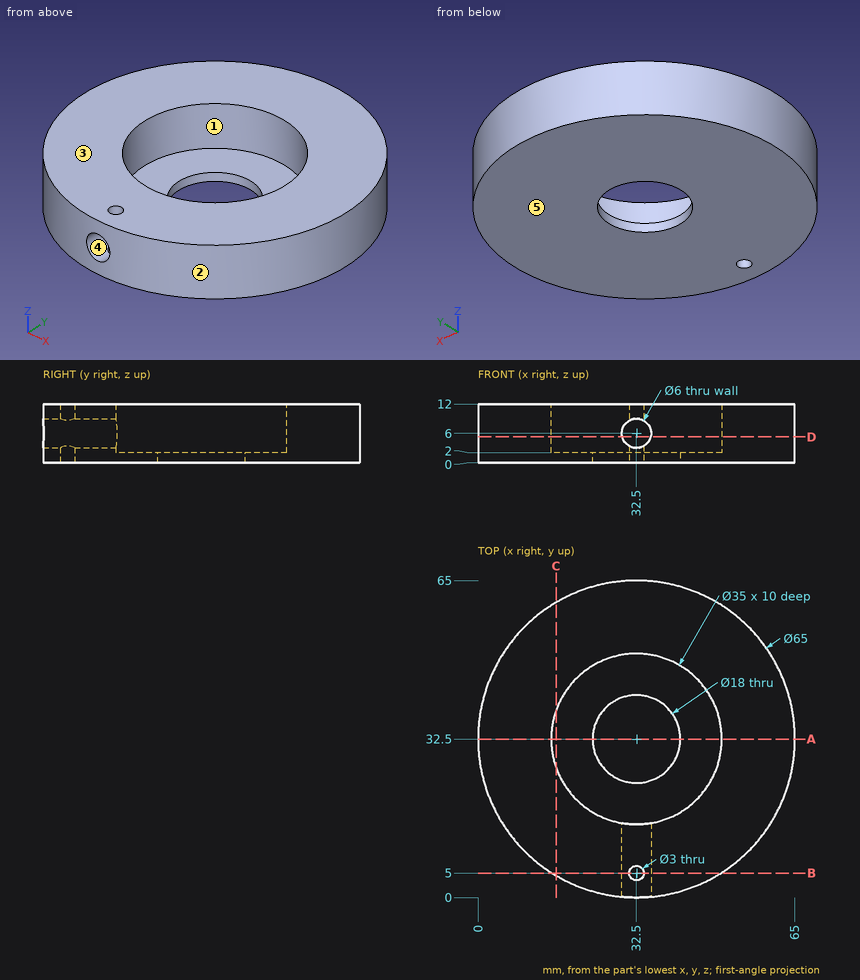
Could you check a few things on this drawing? It's one solid part, dimensions in mm from its lowest x, y, z. A direction names the side the tool comes from. Coordinates: 2 decimals unless noted, no trailing zeros. Write each loop counter-clockwise with the first axis right and the second up, starting at its lowest first coordinate (ties: lowest second). Pieces come first, ordered by that corner, then holes.
1) Thinking about a two-plate mould opening in Z: for the marked faces 3, 4 and 5, which applies, +Z half, -Z half, draft (parallel to the pull), parting line (faces both ways), or undercut?
Filled in:
face 3: +Z half
face 4: undercut
face 5: -Z half
2) Which directions (+Z, -Z, +X, -X, +Y, -Y) give clear straight access to the entire face, cutting with the end or side of a thin tool? Please do the marked faces 1 and 2.
Filled in:
face 1: +Z
face 2: +Z, -Z
3) If we section it at A-A (y = 32.5): List the corners of the cut face in (x, z) for me, plus the area to 3 significant figures.
Filled in:
outline: (0, 0) - (23.5, 0) - (23.5, 2) - (15, 2) - (15, 12) - (0, 12) - close; (41.5, 0) - (65, 0) - (65, 12) - (50, 12) - (50, 2) - (41.5, 2) - close
area: 394 mm2
4) If we section it at D-D (z = 5.25): List the corners of the cut face in (x, y) for me.
Filled in:
outline: (29.6, 0.13) - (29.6, 15.24) arc R17.5 cw (long way) to (35.4, 15.24) - (35.4, 0.13) arc R32.5 ccw (long way) to start
5) I'm going to push flat-ended pins straight in: pin 1 (4 mm diameter, centred on x = 32.5, y = 5, fed in from +Z); pin 2 (5 mm diameter, centred on x = 32.5, z = 6, fed in from +Y); pin 3 (2.5 mm diameter, centred on x = 32.5, y = 5, fed in from +Z); pin 4 (20.5 mm diameter, centred on x = 32.5, y = 32.5, fed in from +Z). Where does each tip first touch, or does it pass through?
Filled in:
pin 1: stops at z = 12
pin 2: stops at y = 65
pin 3: passes through
pin 4: stops at z = 2
6) If I drill on line 1 (Y direction, x = 32.5, z = 2.65); line 2 (X direction, y = 32, z = 8.75); line 3 (Z direction, x = 32.5, y = 9.25), over which ranges is the centre line in solid material (lowest first)?
Filled in:
line 1: y = 0 to 3.5, 6.5 to 15, 50 to 65
line 2: x = 0 to 15.01, 49.99 to 65
line 3: z = 0 to 3, 9 to 12
7) If we section it at C-C (x = 16): List the corners of the cut face in (y, z) for me.
Filled in:
outline: (4.5, 0) - (60.5, 0) - (60.5, 12) - (38.33, 12) - (38.33, 2) - (26.67, 2) - (26.67, 12) - (4.5, 12) - close
8) If we section it at B-B (y = 5): List the corners of the cut face in (x, z) for me, plus the area to 3 significant figures.
Filled in:
outline: (15.18, 0) - (31, 0) - (31, 3.4) arc R3 cw to (31, 8.6) - (31, 12) - (15.18, 12) - close; (34, 0) - (49.82, 0) - (49.82, 12) - (34, 12) - (34, 8.6) arc R3 cw to (34, 3.4) - close
area: 369 mm2
